Design review of the part built by this model. Coordinates are the model's own, in mm. Face numbers are marked on the shaded views. A direction names the side the tool comes from. Coordinates: 2 decimals unless noted, no trailing zeros. Order: outer loops, then holes, each group sorted by start corner. A loop starts at its lowest first (then second) coordinate and runs counter-clockwise, first axis right, second up. Notation, with made-up numbers: (12, 41.25) -> (41, 41.25) arc R34 ccw to (41, 80.25) -> close; hole circle Ø9 at (-35.5, -39.5). An arc over 180 degrees is marked (long way). Use a Markdown table: item, result. Add a question column.
Q1. Wall thickness on probe 1 along Z at (x, y) = (15, 8.25); probe 2 along X at (y, z) = (1.25, 23.5); probe 3 along Z at (x, y) = (0, 0.7): over which ranges is each line inside the solid? List them lowest first.
Q2. Insertion check: pin 1 (8 mm diameter, centred on x = -2, z = 25.5, fed in from -Y); pin 2 (2.5 mm diameter, centred on x = 3.5, y = 0.5, fed in from +Z); pin 3 (4 mm diameter, centred on x = 11.5, z = -3.5, fed in from +Y); pin 4 (1.1 mm diameter, centred on x = 4, y = 1.5, fed in from -Z). Each pin has a flat end and moves straight along its axis. Give the tip position at first contact, or say it passes through.
Q3. Machinability: for the marked faces 1, 2, 3, 4 and 5, which of the approach directions +Z, -Z, +X, -X, +Y, -Y give a long, thin tool a straight path to every point of the face, cutting with its end or side? Answer none if there is none.
Q4. The part is to be moulded in two halves that separate along X. For the marked faces 6, 7, 8 and 9, say which applies: pulls with the +X half, pulls with the -X half, needs draft (parallel to the pull), parting line crosses it, or undercut.
Q5. Add section D-D (z = 13). State the section outline as (x, y) points, then the cut area to 3 significant figures.
Q6. Add section B-B (y = 7.5). State the section outline as (x, z) points, then the cut area to 3 significant figures.
Q7. Add section C-C (z = 0). State the section outline as (x, y) points.
Q8. Add section A-A (x = 0). State the section outline as (y, z) points, then the cut area to 3 significant figures.
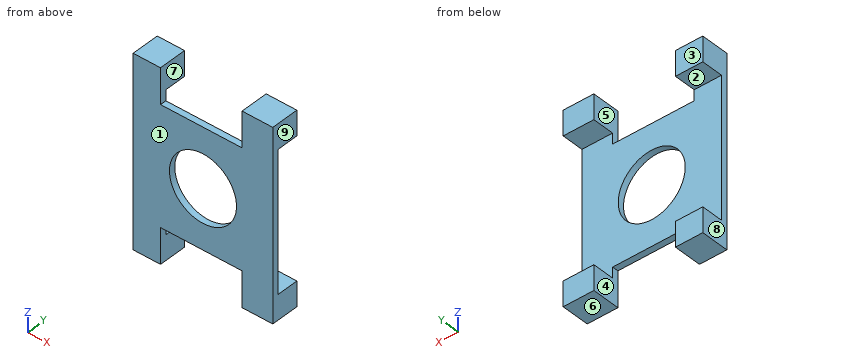
Autodesk Inventor part; units mm, degrees
ref_plane "YZ Plane" through (0, 0, 0) normal (1, 0, 0) x (0, 1, 0)
ref_plane "XZ Plane" through (0, 0, 0) normal (0, 1, 0) x (-1, 0, 0)
ref_plane "XY Plane" through (0, 0, 0) normal (0, 0, 1) x (1, 0, 0)
sketch "Sketch1" plane through (0, 0, 0) normal (0, 1, 0) x (-1, 0, 0)
  circle A0 centre (0, 0) radius 12
  line L0 (25, -21.2) -> (-25, -21.2)
  line L1 (25, -21.2) -> (25, 21.2)
  line L2 (25, 21.2) -> (-25, 21.2)
  line L3 (-25, 21.2) -> (-25, -21.2)
  line L4 (25, 21.2) -> (25, 25)
  line L5 (15.2, 21.2) -> (15.2, 25)
  line L6 (25, -21.2) -> (25, -25)
  line L7 (15.2, -21.2) -> (15.2, -25)
  line L8 (25, -25) -> (15.2, -25)
  line L9 (25, 25) -> (15.2, 25)
  line L10 (-25, 21.2) -> (-25, 25)
  line L11 (-14, 21.2) -> (-14, 25)
  line L12 (-25, -21.2) -> (-25, -25)
  line L13 (-14, -21.2) -> (-14, -25)
  line L14 (-14, -25) -> (-25, -25)
  line L15 (-14, 25) -> (-25, 25)
  point P0 (25, 0)
  point P1 (0, -21.2)
  dimension "d0" = 24
  dimension "d4" = 50
  dimension "d5" = 42.4
  dimension "d8" = 9.8
  dimension "d10" = 50
  dimension "d11" = 11
extrude "Extrusion1" add sketch "Sketch1" along normal blind 2.2
sketch "Sketch2" plane through (0, 0, 0) normal (0, -1, 0) x (1, 0, 0)
  line L0 (25, 25) -> (25, -25) construction
  line L1 (-25, 25) -> (-15.2, 25) construction
  line L2 (-15.2, -25) -> (-25, -25) construction
  line L3 (25, -25) -> (14, -25) construction
  line L4 (-25, 25) -> (-15.2, 25)
  line L5 (-25, -25) -> (-15.2, -25)
  line L6 (25, -25) -> (14, -25) construction
  line L7 (14, -25) -> (25, -25)
  line L8 (14, 25) -> (25, 25) construction
  line L9 (14, 25) -> (25, 25)
  line L10 (-25, 25) -> (-25, 33.89)
  line L11 (-25, 33.89) -> (-15.2, 33.89)
  line L12 (-15.2, 33.89) -> (-15.2, 25)
  line L13 (14, 25) -> (14, 33.89)
  line L14 (14, 33.89) -> (25, 33.89)
  line L15 (25, 33.89) -> (25, 25)
  line L16 (-15.2, -25) -> (-25, -25) construction
  line L17 (-25, -25) -> (-25, -33.89)
  line L18 (-25, -33.89) -> (-15.2, -33.89)
  line L19 (-15.2, -33.89) -> (-15.2, -25)
  line L20 (14, -25) -> (14, -33.89)
  line L21 (14, -33.89) -> (25, -33.89)
  line L22 (25, -33.89) -> (25, -25)
  dimension "d12" = 8.89
  dimension "d13" = 8.89
  dimension "d14" = 8.89
  dimension "d15" = 8.89
extrude "Extrusion2" add sketch "Sketch2" against normal blind 10
properties part number "Cover"
Established:
| question | item | result |
|---|---|---|
| 1 | probe 1 | -33.89 to -25, 25 to 33.89 |
| 1 | probe 2 | -25 to -15.2, 14 to 25 |
| 1 | probe 3 | -21.2 to -12, 12 to 21.2 |
| 2 | pin 1 | through |
| 2 | pin 2 | z = 21.2 |
| 2 | pin 3 | y = 2.2 |
| 2 | pin 4 | z = -21.2 |
| 3 | face 1 | +Z, -Z, +X, -X, -Y |
| 3 | face 2 | +X, -X, +Y |
| 3 | face 3 | +Z, -Z, +X, -X, +Y |
| 3 | face 4 | -Z, +Y, -Y |
| 3 | face 5 | +Z, +Y, -Y |
| 4 | face 6 | needs draft |
| 4 | face 7 | undercut |
| 4 | face 8 | pulls with the -X half |
| 4 | face 9 | pulls with the +X half |
| 5 | outline | (-25, 0) -> (25, 0) -> (25, 2.2) -> (-25, 2.2) -> close |
| 5 | area | 110 mm^2 |
| 6 | outline | (-25, -33.89) -> (-15.2, -33.89) -> (-15.2, -25) -> (-25, -25) -> close; (-25, 25) -> (-15.2, 25) -> (-15.2, 33.89) -> (-25, 33.89) -> close; (14, -33.89) -> (25, -33.89) -> (25, -25) -> (14, -25) -> close; (14, 25) -> (25, 25) -> (25, 33.89) -> (14, 33.89) -> close |
| 6 | area | 370 mm^2 |
| 7 | outline | (-25, 0) -> (-12, 0) -> (-12, 2.2) -> (-25, 2.2) -> close; (12, 0) -> (25, 0) -> (25, 2.2) -> (12, 2.2) -> close |
| 8 | outline | (0, -21.2) -> (2.2, -21.2) -> (2.2, -12) -> (0, -12) -> close; (0, 12) -> (2.2, 12) -> (2.2, 21.2) -> (0, 21.2) -> close |
| 8 | area | 40.5 mm^2 |
